```python
from build123d import *

# Parameters (mm, degrees)
SCHNITT_LINEAR_AUSTRAGEN1_DEPTH = 3
VERRUNDUNG1_R                   = 0.3
KREISMUSTER1_COUNT              = 2
KREISMUSTER1_ANGLE              = 90


with BuildPart() as part:
    # Skizze1 → Rotation1 (revolve)
    with BuildSketch(Plane(origin=(0, 0, 0), x_dir=(0, 0, -1), z_dir=(0, 1, 0))):
        Polygon((0, 0), (0, 24), (4, 24), (4, 20), (2.25, 20), (2.25, 0), align=None)
    revolve(axis=Axis((0, 0, 0), (-1, 0, 0)))

    # Skizze2 → Schnitt-Linear austragen1 (cut)
    with BuildSketch(Plane(origin=(-24, 0, 0), x_dir=(0, 1, 0), z_dir=(-1, 0, 0))):
        Polygon((0, 2.886751346), (-2.5, 1.443375673), (-2.5, -1.443375673), (0, -2.886751346), (2.5, -1.443375673), (2.5, 1.443375673), align=None)
    extrude(amount=-SCHNITT_LINEAR_AUSTRAGEN1_DEPTH, mode=Mode.SUBTRACT)

    # Verrundung1
    verrundung1_edges = [part.edges().sort_by_distance(p)[0] for p in [
        (-20, 0, 2.25),
        (-20, 0, 4),
        (-24, 0, 4),
    ]]
    fillet(verrundung1_edges, radius=VERRUNDUNG1_R)


with BuildPart() as kreismuster1_1:
    # Kreismuster1: pattern copy
    add(part.part.rotate(Axis((0, 0, 0), (0, -1, 0)), 1 * KREISMUSTER1_ANGLE / (KREISMUSTER1_COUNT - 1)))


solid = kreismuster1_1.part
```
Can you work these out from the model? Positions are in its coordinate system, mm. A direction names the side the tool comes from. Give positions to 0.01 mm unless a question says otherwise; leave off trailing zeros. Order: outer loops, then holes, each group sorted by start corner. A loop starts at its lowest first (then second) coordinate and runs counter-clockwise, first axis right, second up. Notation, with made-up numbers: (31.25, 2) - (44.25, 2) arc R20 cw to (44.25, 12) - close; hole circle Ø11 at (-28.75, 44). An arc over 180 degrees is marked (long way). Use a Markdown table: item, result. Add a question column.
Q1. If we mould it in two halves opening along Y, with no side actions, what happens to faces 4 (the cylindrical face through (-0.867, 3.905, -21.976)), 5 (the flat face through (1, -3, -20)), 6 (the flat face through (2.155, 1.267, -22.521))? For each: released by +Y, released by -Y, zero draft, split by the parting line, or undercut.
Q2. I'm going to push flat-ended pins straight in: pin 1 (1 mm diameter, centred on y = 2.5, z = -17.5, fed in from -X); pin 2 (4 mm diameter, centred on x = 0, z = -15.5, fed in from +Y); pin 3 (1.5 mm diameter, centred on y = -1, z = -5.5, fed in from +X); pin 4 (3 mm diameter, centred on x = 0.5, z = -23, fed in from +Y). Where does each tip first touch, or does it pass through?
Q3. On a 3-axis mill with a long thin cutter (end or side, diameter ignored), from which of +Z, -Z, +X, -X, +Y, -Y can I reach the whole of each face in a straight line? I mean faces 1 (the cylindrical face through (-0.29, -2.23, -9.71)), 2 (the flat face through (0, 0, -21)), 3 (the flat face through (0, 0, 0)). Say none if no direction works.
Q4. If we section it at B-B on z = -10: Write out the boundary of the cut face in (x, y), plus the area to 3 significant figures.
Q5. If we section it at A-A on x = 0: Write out the boundary of the cut face in (y, z).
Q6. Please list where these lines run through material, in increasing order: line 1 along Z through (x, y) = (0.5, 1); line 2 along Z through (x, y) = (-2.25, 2); line 3 along X through (y, z) = (0, -6.75).
Answers follow:
| question | item | result |
|---|---|---|
| 1 | face 4 | split by the parting line |
| 1 | face 5 | zero draft |
| 1 | face 6 | undercut |
| 2 | pin 1 | stops at x = -1.03 |
| 2 | pin 2 | stops at y = 2.25 |
| 2 | pin 3 | stops at x = 2.24 |
| 2 | pin 4 | stops at y = 4 |
| 3 | face 1 | +Z |
| 3 | face 2 | -Z |
| 3 | face 3 | +Z, +X, -X, +Y, -Y |
| 4 | outline | circle Ø4.5 at (0, 0) |
| 4 | area | 15.9 mm^2 |
| 5 | outline | (-4, -23.7) arc R0.3 ccw to (-3.7, -24) - (-2.5, -24) - (-2.5, -21) - (2.5, -21) - (2.5, -24) - (3.7, -24) arc R0.3 ccw to (4, -23.7) - (4, -20.3) arc R0.3 ccw to (3.7, -20) - (2.55, -20) arc R0.3 cw to (2.25, -19.7) - (2.25, 0) - (-2.25, 0) - (-2.25, -19.7) arc R0.3 cw to (-2.55, -20) - (-3.7, -20) arc R0.3 ccw to (-4, -20.3) - close |
| 6 | line 1 | z = -21 to 0 |
| 6 | line 2 | z = -24 to -20 |
| 6 | line 3 | x = -2.25 to 2.25 |
